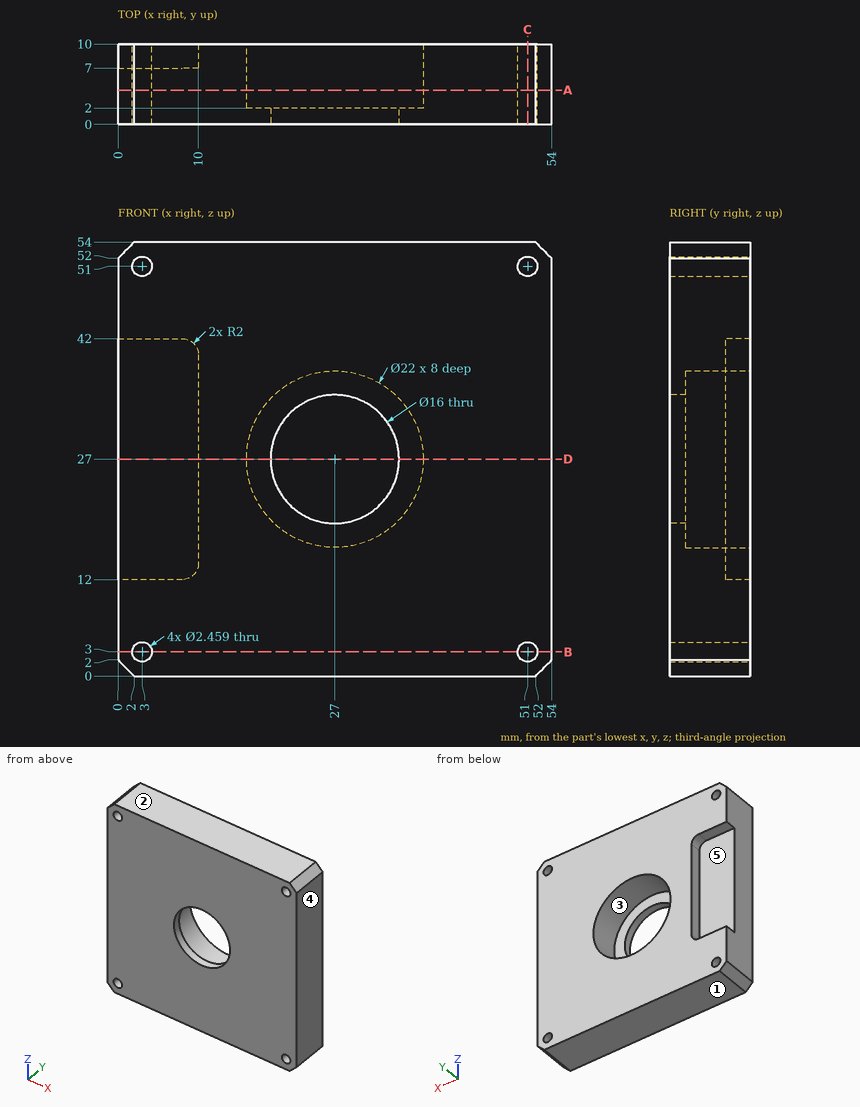
Verification items for this drawing (mm, ordinates from the low corner). A direction names the side the tool comes from. Round coordinates to 2 decimals unless told otherwise and drop trailing zeros. Order: outer loops, then holes, each group sorted by start corner. A loop starts at its lowest first (then second) coordinate and runs counter-clockwise, first axis right, second up. Notation, with made-up numbers: (13.25, -4) - (56.25, -4) arc R18 cw to (56.25, 9) - close; hole circle Ø7 at (62, 4). An arc over 180 degrees is marked (long way). Use CSV: the item, a comma, the result in double quotes.
(1) Section check D-D on z = 27. Record the boundary of the cut face in (x, y).
Entries:
outline,"(0, 0) - (19, 0) - (19, 2) - (16, 2) - (16, 10) - (10, 10) - (10, 7) - (0, 7) - close; (35, 0) - (54, 0) - (54, 10) - (38, 10) - (38, 2) - (35, 2) - close"
(2) Mould release check, pull along Z, two halves, no side actions. Record for the marked faces 1, 2 and 3: released by +Z, released by -Z, zero draft, split by the parting line, or undercut.
Entries:
face 1,"released by -Z"
face 2,"released by +Z"
face 3,"undercut"
(3) Section check B-B on z = 3. Record the boundary of the cut face in (x, y).
Entries:
outline,"(0, 0) - (1.77, 0) - (1.77, 10) - (0, 10) - close; (4.23, 0) - (49.77, 0) - (49.77, 10) - (4.23, 10) - close; (52.23, 0) - (54, 0) - (54, 10) - (52.23, 10) - close"
(4) Thickness scan on probe 1 along X at (y, z) = (4.25, 3); probe 2 along Z at (x, y) = (3, 8). Record the ranges inside material, lowest first. Write a range as from..to.
Entries:
probe 1,"0..1.77, 4.23..49.77, 52.23..54"
probe 2,"0..1.77, 4.23..12, 42..49.77, 52.23..54"
(5) Section check A-A on y = 4.25. Record the boundary of the cut face in (x, z).
Entries:
outline,"(0, 2) - (2, 0) - (52, 0) - (54, 2) - (54, 52) - (52, 54) - (2, 54) - (0, 52) - close; hole circle Ø2.46 at (3, 3); hole circle Ø2.46 at (3, 51); hole circle Ø22 at (27, 27); hole circle Ø2.46 at (51, 3); hole circle Ø2.46 at (51, 51)"
(6) Gauge pin test, flat ends, axial feed: pin 1 Ø8 at (x, z) = (30, 32) entering from -Y; pin 2 Ø8 at (x, z) = (3.5, 30) entering from +Y. Record the tip position at first contact, or that the pin passes through.
Entries:
pin 1,"y = 0"
pin 2,"y = 7"
(7) Section check C-C on x = 51. Record the boundary of the cut face in (y, z).
Entries:
outline,"(0, 0) - (10, 0) - (10, 1.77) - (0, 1.77) - close; (0, 4.23) - (10, 4.23) - (10, 49.77) - (0, 49.77) - close; (0, 52.23) - (10, 52.23) - (10, 54) - (0, 54) - close"
(8) Access from +Z, -Z, +X, -X, +Y, -Y to the whole of each face (thin tool, end or side, straight path). Record for the marked faces 4 and 5.
Entries:
face 4,"+Z, -Z, +X, +Y, -Y"
face 5,"-X, +Y"
